CAD build for the part. Positions are in the model's coordinates, mm. Face numbers are marked on the shaded views. Round coordinates to 2 decimals unless told otherwise and drop trailing zeros. Loops run counter-clockwise (first coordinate to the right, second up) from the corner with the lowest first, then second, coordinate; pieces in that order, holes last.
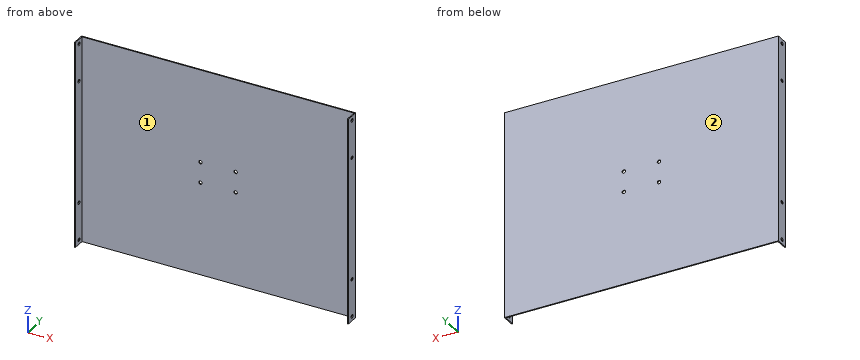
```python
from build123d import *

# Parameters (mm, degrees)
ESBO_O1_W                  = 320
ESBO_O1_H                  = 240
RESSALTO_EXTRUS_O1_DEPTH   = 15
ESBO_O2_W                  = 317.6
ESBO_O2_H                  = 240
CORTE_EXTRUS_O1_DEPTH      = 13.8
CORTE_EXTRUS_O2_START      = 10
ESBO_O3_R                  = 2
CORTE_EXTRUS_O2_DEPTH      = 13.8
CORTE_EXTRUS_O3_DEPTH      = 170
CORTE_EXTRUS_O3_DEPTH_BACK = 170
ESBO_O4_R                  = 2


with BuildPart() as part:
    # Esboço1 → Ressalto-extrusão1 (new body)
    with BuildSketch(Plane(origin=(0, 0, 0), x_dir=(1, 0, 0), z_dir=(0, 1, 0))):
        Rectangle(ESBO_O1_W, ESBO_O1_H)
    extrude(amount=RESSALTO_EXTRUS_O1_DEPTH)

    # Esboço2 → Corte-extrusão1 (cut)
    with BuildSketch(Plane(origin=(0, 0, 0), x_dir=(1, 0, 0), z_dir=(0, 1, 0))):
        Rectangle(ESBO_O2_W, ESBO_O2_H)
    extrude(amount=CORTE_EXTRUS_O1_DEPTH, mode=Mode.SUBTRACT)

    # Esboço3 → Corte-extrusão2 (cut)
    with BuildSketch(Plane(origin=(0, 0, 0), x_dir=(1, 0, 0), z_dir=(0, 1, 0)).offset(CORTE_EXTRUS_O2_START)):
        with Locations(Location((-20.52, -12, 0), (0, 0, 90))):
            Circle(ESBO_O3_R)
        with Locations(Location((20.52, -12, 0), (0, 0, 90))):
            Circle(ESBO_O3_R)
        with Locations(Location((20.52, 12, 0), (0, 0, 90))):
            Circle(ESBO_O3_R)
        with Locations(Location((-20.52, 12, 0), (0, 0, 90))):
            Circle(ESBO_O3_R)
    extrude(amount=CORTE_EXTRUS_O2_DEPTH, mode=Mode.SUBTRACT)

    # Esboço4 → Corte-extrusão3 (cut, two sides: drawn at the far end of the back side and taken through both)
    with BuildSketch(Plane(origin=(0, 0, 0), x_dir=(0, 0, -1), z_dir=(1, 0, 0)).offset(-CORTE_EXTRUS_O3_DEPTH_BACK)):
        with Locations((114.8, 7.5)):
            Circle(ESBO_O4_R)
        with Locations((71.2, 7.5)):
            Circle(ESBO_O4_R)
        with Locations((-114.8, 7.5)):
            Circle(ESBO_O4_R)
        with Locations((-71.2, 7.5)):
            Circle(ESBO_O4_R)
    extrude(amount=CORTE_EXTRUS_O3_DEPTH + CORTE_EXTRUS_O3_DEPTH_BACK, mode=Mode.SUBTRACT)


solid = part.part
```
Item 1: Two-plate mould, pull along X, no slides. Class the marked faces 1 and 2: released by +X, released by -X, zero draft, split by the parting line, or undercut.
Answers follow:
face 1: undercut
face 2: zero draft
Item 2: Cut at B-B, the plane x = 46. Give the cut face in (y, z), plus the area to 3 significant figures.
Answers follow:
outline: (13.8, -120) - (15, -120) - (15, 120) - (13.8, 120) - close
area: 288 mm2
Item 3: Probe line 1 (Z direction, x = -159.15, y = 7.5); line 2 (Y direction, x = 159.6, z = 71.2); line 3 (X direction, y = 10, z = -56). List the from-to ranges inside material, lowest first.
Answers follow:
line 1: z = -120 to -116.8, -112.8 to -73.2, -69.2 to 69.2, 73.2 to 112.8, 116.8 to 120
line 2: y = 0 to 5.5, 9.5 to 15
line 3: x = -160 to -158.8, 158.8 to 160
Item 4: Cut at A-A, the plane z = -47. Give the cut face in (x, y).
Answers follow:
outline: (-160, 0) - (-158.8, 0) - (-158.8, 13.8) - (158.8, 13.8) - (158.8, 0) - (160, 0) - (160, 15) - (-160, 15) - close
Item 5: Flat gauge pins, fed straight in: P1, Ø2.5, axis at y = 7.5, z = -71.2, coming from the -X side; P2, Ø5, axis at x = 20.52, z = 12, coming from the -Y side. Where does each tip first touch, or does it go through?
Answers follow:
P1: passes through
P2: stops at y = 13.8
